```python
from build123d import *

# Parameters (mm, degrees)
SKETCH1_R               = 36
BOSS_EXTRUDE1_DEPTH     = 50
SKETCH2_R               = 23
CUT_EXTRUDE1_DEPTH      = 22
SKETCH3_R               = 14
CUT_EXTRUDE2_DEPTH      = 22
SKETCH4_R               = 15.25
CUT_EXTRUDE3_DEPTH      = 6
SKETCH5_W               = 1.25
SKETCH5_H               = 1.75
CUT_EXTRUDE4_DEPTH      = 72.3582511
CUT_EXTRUDE4_DEPTH_BACK = 72.3582511
SKETCH6_R               = 3
CHAMFER1_SIZE           = 1


with BuildPart() as part:
    # Sketch1 → Boss-Extrude1 (new body)
    with BuildSketch(Plane(origin=(0, 0, 0), x_dir=(1, 0, 0), z_dir=(0, 1, 0))):
        with Locations(Location((0, 0, 0), (0, 0, 270))):
            Circle(SKETCH1_R)
    extrude(amount=BOSS_EXTRUDE1_DEPTH)

    # Sketch2 → Cut-Extrude1 (cut)
    with BuildSketch(Plane(origin=(0, 50, 0), x_dir=(1, 0, 0), z_dir=(0, 1, 0))):
        with Locations(Location((0, 0, 0), (0, 0, 270))):
            Circle(SKETCH2_R)
    extrude(amount=-CUT_EXTRUDE1_DEPTH, mode=Mode.SUBTRACT)

    # Sketch3 → Cut-Extrude2 (cut)
    with BuildSketch(Plane.XZ):
        with Locations(Location((0, 0, 0), (0, 0, 270))):
            Circle(SKETCH3_R)
    extrude(amount=-CUT_EXTRUDE2_DEPTH, mode=Mode.SUBTRACT)

    # Sketch4 → Cut-Extrude3 (cut)
    with BuildSketch(Plane(origin=(0, 28, 0), x_dir=(1, 0, 0), z_dir=(0, 1, 0))):
        with Locations(Location((0, 0, 0), (0, 0, 270))):
            Circle(SKETCH4_R)
    extrude(amount=-CUT_EXTRUDE3_DEPTH, mode=Mode.SUBTRACT)

    # Sketch5 → Cut-Revolve1 (revolve, cut)
    with BuildSketch(Plane.XY, mode=Mode.PRIVATE) as cut_revolve1_sk:
        with Locations((23.625, 46)):
            Rectangle(SKETCH5_W, SKETCH5_H)
    revolve(cut_revolve1_sk.sketch.rotate(Axis((0, 0, 0), (0, 1, 0)), 270), axis=Axis((0, 0, 0), (0, 1, 0)), mode=Mode.SUBTRACT)

    # Sketch6 → Cut-Extrude4 (cut, two sides: drawn at the far end of the back side and taken through both)
    with BuildSketch(Plane.XY.offset(-CUT_EXTRUDE4_DEPTH_BACK)):
        with Locations((0, 11)):
            Circle(SKETCH6_R)
    extrude(amount=CUT_EXTRUDE4_DEPTH + CUT_EXTRUDE4_DEPTH_BACK, mode=Mode.SUBTRACT)

    # Chamfer1
    chamfer1_edges = [part.edges().sort_by_distance(p)[0] for p in [
        (0, 0, -36),
        (0, 50, -36),
    ]]
    chamfer(chamfer1_edges, length=CHAMFER1_SIZE)


solid = part.part
```
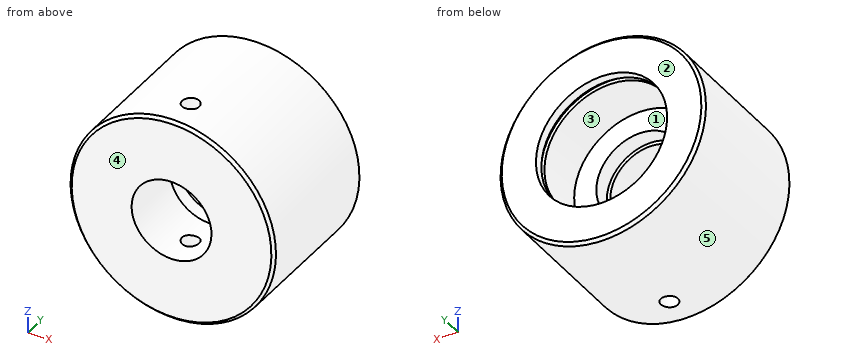
For this review, take the finished solid that the model builds, in its own axes (mm). Face numbers are marked on the shaded views. A direction names the side the tool comes from. Coordinates: 2 decimals unless noted, no trailing zeros. Order: outer loops, then holes, each group sorted by start corner. A loop starts at its lowest first (then second) coordinate and runs counter-clockwise, first axis right, second up. Notation, with made-up numbers: (27.5, 60) -> (33.5, 60) arc R21 ccw to (33.5, 97) -> close; hole circle Ø9 at (69, 85). An arc over 180 degrees is marked (long way). Answer as CSV lines item,"result".
Q1. Clearance check with flat-ended pins moving along their axes: pin 1 Ø1 at (y, z) = (41, 10.5) entering from -X; pin 2 Ø12 at (y, z) = (43, 20) entering from +X; pin 3 Ø1 at (y, z) = (23.5, 8.5) entering from -X. State where each tip first meets the part, or that it passes through.
Model answer:
pin 1,"stops at x = -34.58"
pin 2,"stops at x = 33.17"
pin 3,"stops at x = -35.1"
Q2. We need section B-B (y = 11). State the section outline as (x, z) points.
Model answer:
outline,"(-3, -35.87) -> (-3, -13.67) arc R14 cw to (-3, 13.67) -> (-3, 35.87) arc R36 ccw to start; (3, -35.87) arc R36 ccw to (3, 35.87) -> (3, 13.67) arc R14 cw to (3, -13.67) -> close"
Q3. Wall thickness on line 1 along X through (y, z) = (25.25, 0); line 2 along Y through (x, z) = (4.5, -23.5) (3 decimals); line 3 along X through (y, z) = (46, 0): over which ranges is each line inside the solid? List them lowest first. Write a range as [from, to].
Model answer:
line 1,"x = [-36, -15.25], [15.25, 36]"
line 2,"y = [0, 45.125], [46.875, 50]"
line 3,"x = [-36, -24.25], [24.25, 36]"
Q4. We need section C-C (x = 0). Count the separate pieces of the cut face and the enclosed holes in it, plus the area to 3 significant figures.
Model answer:
separate pieces,"4"
enclosed holes,"0"
area,"1,520 mm2"
Q5. For the marked faces 1 and 2, list the 3-axis set-ups (+Z, -Z, +X, -X, +Y, -Y) from which the entire face can be reached by the end or side of a thin tool; tool diameter is ignored.
Model answer:
face 1,"+Y"
face 2,"+Z, -Z, +X, -X, +Y"
Q6. Draft analysis for pull direction X (two halves, no side actions). For the marked faces 3, 4 and 5, state which applies: released by +X, released by -X, zero draft, split by the parting line, or undercut.
Model answer:
face 3,"undercut"
face 4,"zero draft"
face 5,"split by the parting line"
Q7. We need section D-D (y = 23.5). State the section outline as (x, z) points.
Model answer:
outline,"circle Ø72 at (0, 0); hole circle Ø30.5 at (0, 0)"
Q8. We need section A-A (z = 0). State the section outline as (x, y) points (3 decimals), plus the area to 3 significant figures.
Model answer:
outline,"(-36, 1) -> (-35, 0) -> (-14, 0) -> (-14, 22) -> (-15.25, 22) -> (-15.25, 28) -> (-23, 28) -> (-23, 45.125) -> (-24.25, 45.125) -> (-24.25, 46.875) -> (-23, 46.875) -> (-23, 50) -> (-35, 50) -> (-36, 49) -> close; (14, 0) -> (35, 0) -> (36, 1) -> (36, 49) -> (35, 50) -> (23, 50) -> (23, 46.875) -> (24.25, 46.875) -> (24.25, 45.125) -> (23, 45.125) -> (23, 28) -> (15.25, 28) -> (15.25, 22) -> (14, 22) -> close"
area,"1,780 mm2"
